Could you check a few things on this drawing? It's one solid part, dimensions in mm from its lowest x, y, z. Coordinates: 2 decimals unless noted, no trailing zeros. Write each loop counter-clockwise with the first axis right and the second up, starting at its lowest first coordinate (ties: lowest second). Pieces come first, ordered by that corner, then holes.
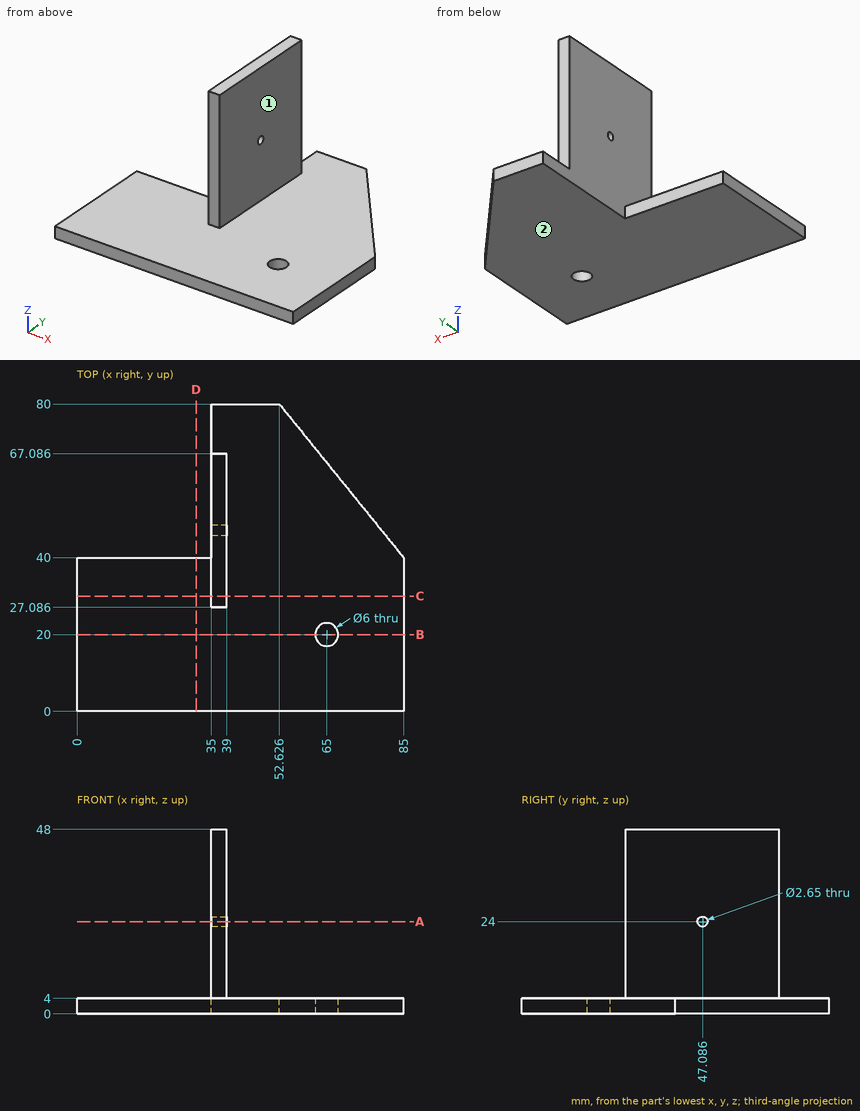
1) Imagine slicing it at A-A on z = 24. Please give me the cut outline in (x, y) (1 decimal), then the cut area to 3 significant figures.
Values follow:
outline: (35, 27.1) - (39, 27.1) - (39, 45.8) - (35, 45.8) - close; (35, 48.4) - (39, 48.4) - (39, 67.1) - (35, 67.1) - close
area: 149 mm2
2) Imagine slicing it at C-C on y = 30. Please give me the cut outline in (x, z), then the cut area to 3 significant figures.
Values follow:
outline: (0, 0) - (85, 0) - (85, 4) - (39, 4) - (39, 48) - (35, 48) - (35, 4) - (0, 4) - close
area: 516 mm2
3) Imagine slicing it at B-B on y = 20. Please give me the cut outline in (x, z).
Values follow:
outline: (0, 0) - (62, 0) - (62, 4) - (0, 4) - close; (68, 0) - (85, 0) - (85, 4) - (68, 4) - close
4) Will these pins go through, and if not, where does the flat tip stop? pin 1 (3 mm diameter, centred on y = 47.09, z = 24, fed in from +X); pin 2 (3.5 mm diameter, centred on x = 65, y = 20, fed in from -Z); pin 3 (14.5 mm diameter, centred on y = 50.5, z = 24, fed in from -X); pin 4 (2 mm diameter, centred on x = 36.5, z = 19, fed in from +Y).
Values follow:
pin 1: stops at x = 39
pin 2: passes through
pin 3: stops at x = 35
pin 4: stops at y = 67.09
5) I need wall thicknesses on probe 1 along X at (y, z) = (44.5, 13); probe 2 along Y at (x, z) = (37, 24) (1 decimal); probe 3 along Z at (x, y) = (49.5, 7). Which ranges of each line are inside material? Lowest first, please.
Values follow:
probe 1: x = 35 to 39
probe 2: y = 27.1 to 45.8, 48.4 to 67.1
probe 3: z = 0 to 4
6) Imagine slicing it at D-D on x = 31. Please give me the cut outline in (y, z), then the cut area to 3 significant figures.
Values follow:
outline: (0, 0) - (40, 0) - (40, 4) - (0, 4) - close
area: 160 mm2
7) We'd pull the mould along X, two halves only. Please class the marked faces 1 and 2: pulls with the +X half, pulls with the -X half, needs draft (parallel to the pull), parting line crosses it, or undercut.
Values follow:
face 1: pulls with the +X half
face 2: needs draft
